Work out the finished part from the listing and answer in its coordinate system (mm). A direction names the side the tool comes from. Round coordinates to 2 decimals unless told otherwise and drop trailing zeros. Loops run counter-clockwise (first coordinate to the right, second up) from the corner with the lowest first, then second, coordinate; pieces in that order, holes last. Notation, with made-up numbers: M -8.5,18.25 L 25.5,18.25 A22 cw 25.5,55.25 Z; hole C 25.25,85 d10. An arc over 180 degrees is marked long. One line per item, written item: value.
```python
from build123d import *

# Parameters (mm, degrees)
BOSS_EXTRUDE1_DEPTH            = 8
CUT_EXTRUDE1_DEPTH             = 7
SKETCH3_R                      = 11
BOSS_EXTRUDE2_DEPTH            = 2
SKETCH4_R                      = 12.925
BOSS_EXTRUDE3_DEPTH            = 8
SKETCH5_R                      = 8.025
CUT_EXTRUDE2_DEPTH             = 31.757112998
SKETCH6_R                      = 6.125
CUT_EXTRUDE3_DEPTH             = 32.032241298
M8_CLEARANCE_HOLE1_D           = 9.25
M8_CLEARANCE_HOLE1_DEPTH       = 11
F_2_5_2_5_DIAMETER_HOLE1_D     = 2.5
F_2_5_2_5_DIAMETER_HOLE1_DEPTH = 10
FILLET1_R                      = 0.150000001
FILLET2_R                      = 0.5
CHAMFER1_SIZE                  = 0.5
CHAMFER1_SIZE2                 = 1
CHAMFER2_SIZE                  = 0.25
CHAMFER3_SIZE                  = 0.25


with BuildPart() as part:
    # Sketch1 → Boss-Extrude1 (new body)
    with BuildSketch(Plane.XZ):
        with BuildLine():
            Line((16.171038928, 21), (-16.171038928, 21))
            ThreePointArc((-16.171038928, 21), (-16.861657425, 20.876977915), (-17.467314594, 20.523046092))
            ThreePointArc((-17.467314594, 20.523046092), (-19.056527753, 19.056527753), (-20.523046092, 17.467314594))
            ThreePointArc((-20.523046092, 17.467314594), (-20.876977915, 16.861657425), (-21, 16.171038928))
            Line((-21, 16.171038928), (-21, -16.171038928))
            ThreePointArc((-21, -16.171038928), (-20.876977915, -16.861657425), (-20.523046092, -17.467314594))
            ThreePointArc((-20.523046092, -17.467314594), (-19.056527753, -19.056527753), (-17.467314594, -20.523046092))
            ThreePointArc((-17.467314594, -20.523046092), (-16.861657425, -20.876977915), (-16.171038928, -21))
            Line((-16.171038928, -21), (16.171038928, -21))
            ThreePointArc((16.171038928, -21), (16.861657424, -20.876977915), (17.467314593, -20.523046092))
            ThreePointArc((17.467314593, -20.523046092), (19.056527753, -19.056527753), (20.523046092, -17.467314593))
            ThreePointArc((20.523046092, -17.467314593), (20.876977914, -16.861657425), (21, -16.171038928))
            Line((21, -16.171038928), (21, 16.171038928))
            ThreePointArc((21, 16.171038928), (20.876977914, 16.861657425), (20.523046092, 17.467314593))
            ThreePointArc((20.523046092, 17.467314593), (19.056527753, 19.056527753), (17.467314593, 20.523046092))
            ThreePointArc((17.467314593, 20.523046092), (16.861657424, 20.876977915), (16.171038928, 21))
        make_face()
    extrude(amount=-BOSS_EXTRUDE1_DEPTH)

    # Sketch2 → Cut-Extrude1 (cut)
    with BuildSketch(Plane.XZ):
        Polygon((-19.5, 8.077164467), (-19.5, -8.077164467), (-8.077164467, -19.5), (8.077164467, -19.5), (19.5, -8.077164467), (19.5, 8.077164467), (8.077164467, 19.5), (-8.077164467, 19.5), align=None)
    extrude(amount=-CUT_EXTRUDE1_DEPTH, mode=Mode.SUBTRACT)

    # Sketch3 → Boss-Extrude2 (add)
    with BuildSketch(Plane(origin=(0, 8, 0), x_dir=(-1, 0, 0), z_dir=(0, 1, 0))):
        with Locations(Location((0, 0, 0), (0, 0, 270))):
            Circle(SKETCH3_R)
    extrude(amount=BOSS_EXTRUDE2_DEPTH)

    # Sketch4 → Boss-Extrude3 (add)
    with BuildSketch(Plane.XZ.offset(-7)):
        with Locations(Location((0, 0, 0), (0, 0, 270))):
            Circle(SKETCH4_R)
    extrude(amount=BOSS_EXTRUDE3_DEPTH)

    # Sketch5 → Cut-Extrude2 (cut, through all)
    with BuildSketch(Plane(origin=(0, 7, 0), x_dir=(1, 0, 0), z_dir=(0, 1, 0))):
        with Locations(Location((0, 0, 0), (0, 0, 90))):
            Circle(SKETCH5_R)
    extrude(amount=-CUT_EXTRUDE2_DEPTH, mode=Mode.SUBTRACT)

    # Sketch6 → Cut-Extrude3 (cut, through all)
    with BuildSketch(Plane(origin=(0, 8, 0), x_dir=(1, 0, 0), z_dir=(0, 1, 0))):
        with Locations(Location((0, 0, 0), (0, 0, 90))):
            Circle(SKETCH6_R)
    extrude(amount=-CUT_EXTRUDE3_DEPTH, mode=Mode.SUBTRACT)

    # M8 Clearance Hole1
    with Locations(Plane(origin=(0, 10, 0), x_dir=(1, 0, 0), z_dir=(0, 1, 0))):
        with Locations((0, 0)):
            Hole(M8_CLEARANCE_HOLE1_D / 2, depth=M8_CLEARANCE_HOLE1_DEPTH)

    # Ø2.5 (2.5) Diameter Hole1
    with Locations(Plane(origin=(0, 0, 0), x_dir=(-1, 0, 0), z_dir=(0, -1, 0))):
        with Locations((15.5, 15.5), (-15.5, -15.5), (-15.5, 15.5), (15.5, -15.5)):
            Hole(F_2_5_2_5_DIAMETER_HOLE1_D / 2, depth=F_2_5_2_5_DIAMETER_HOLE1_DEPTH)

    # Fillet1
    fillet1_edges = [part.edges().sort_by_distance(p)[0] for p in [
        (0, 8, 11),
        (0, 7, 12.925),
    ]]
    fillet(fillet1_edges, radius=FILLET1_R)

    # Fillet2
    fillet2_edges = [part.edges().sort_by_distance(p)[0] for p in [
        (-19.5, 3.5, 8.077164467),
        (-8.077164467, 3.5, 19.5),
        (8.077164467, 3.5, 19.5),
        (19.5, 3.5, 8.077164467),
        (19.5, 3.5, -8.077164467),
        (8.077164467, 3.5, -19.5),
        (-8.077164467, 3.5, -19.5),
        (-19.5, 3.5, -8.077164467),
    ]]
    fillet(fillet2_edges, radius=FILLET2_R)

    # Chamfer1
    chamfer1_edges = [part.edges().sort_by_distance(p)[0] for p in [
        (0, -1, 8.025),
    ]]
    chamfer1_side = [part.faces().sort_by_distance(p)[0] for p in [
        (0, -1, 12.559425794),
    ]]
    chamfer(chamfer1_edges, length=CHAMFER1_SIZE, length2=CHAMFER1_SIZE2, reference=chamfer1_side[0])

    # Chamfer2
    chamfer2_edges = [part.edges().sort_by_distance(p)[0] for p in [
        (16.861657424, 8, 20.876977915),
        (0, 8, 21),
        (-16.861657425, 8, 20.876977915),
        (-19.056527753, 8, 19.056527753),
        (-20.876977915, 8, 16.861657425),
        (-21, 8, 0),
        (-20.876977915, 8, -16.861657425),
        (-19.056527753, 8, -19.056527753),
        (-16.861657425, 8, -20.876977915),
        (0, 8, -21),
        (20.876977914, 8, 16.861657425),
        (16.861657424, 8, -20.876977915),
        (19.056527753, 8, -19.056527753),
        (20.876977914, 8, -16.861657425),
        (21, 8, 0),
        (19.056527753, 8, 19.056527753),
    ]]
    chamfer(chamfer2_edges, length=CHAMFER2_SIZE)

    # Chamfer3
    chamfer3_edges = [part.edges().sort_by_distance(p)[0] for p in [
        (0, 10, 11),
        (0, -1, 12.925),
        (0, 7, 6.125),
        (4.625, 10, 0),
    ]]
    chamfer(chamfer3_edges, length=CHAMFER3_SIZE)


solid = part.part
```
1) Find section A-A (y = 6.25). Give the number of separate pieces and of enclosed holes in the cut face, then the cut area to 3 significant figures.
Check values:
separate pieces: 2
enclosed holes: 6
area: 775 mm2
2) For faces 1 (the face through (-16.421, 4.056, -16.345)), 2 (the face through (13.711, 3.451, -13.866)), 3 (the face through (10.74, 8.94, 2.38)), determine the directions among +Z, -Z, +X, -X, +Y, -Y from which every point of the face is accessible in a straight line to the end or side of a thin tool.
Check values:
face 1: +Y, -Y
face 2: -Y
face 3: +Y
3) Each of these flat-tipped pins is pushed along its axis until it touches: pin 1 (10 mm diameter, centred on x = 2, z = 2, fed in from -Y); pin 2 (3 mm diameter, centred on x = -15.5, z = 15.5, fed in from -Y). Where does it stop, or does it pass through?
Check values:
pin 1: y = 7
pin 2: y = 0
4) Find section B-B (x = -15.5). Give the vertices of the cut face in (y, z).
Check values:
outline: M 0,-21 L 7.75,-21 L 8,-20.75 L 8,-16.75 L 0,-16.75 Z; M 0,-14.25 L 8,-14.25 L 8,14.25 L 0,14.25 L 0,12.08 L 7,12.08 L 7,-12.08 L 0,-12.08 Z; M 0,16.75 L 8,16.75 L 8,20.75 L 7.75,21 L 0,21 Z
5) Find section C-C (z = 15). Give the vertices of the cut face in (x, y).
Check values:
outline: M -21,0 L -16.65,0 L -16.65,8 L -20.75,8 L -21,7.75 Z; M -14.35,0 L -12.58,0 L -12.58,7 L 12.58,7 L 12.58,0 L 14.35,0 L 14.35,8 L -14.35,8 Z; M 16.65,0 L 21,0 L 21,7.75 L 20.75,8 L 16.65,8 Z
6) The mould has two halves that part along X. Classify faces 4 (the face through (-20.874, 3.821, 16.871)), 5 (the face through (-0.3, 7, 13.3)), 6 (the face through (14, 0, 14)): +X half, -X half, draft (parallel to the pull), parting line (faces both ways), or undercut.
Check values:
face 4: -X half
face 5: undercut
face 6: draft
7) Find the intervals of material crossed by probe 1 along X at (y, z) = (2.75, 0) (3 decimals); probe 2 along X at (y, z) = (4.75, 3.5); probe 3 along X at (y, z) = (2, 11), in increasing order. Write a range as from..to.
Check values:
probe 1: -21..-19.5, -12.925..-8.025, 8.025..12.925, 19.5..21
probe 2: -21..-19.5, -12.44..-7.22, 7.22..12.44, 19.5..21
probe 3: -21..-16.58, -6.79..6.79, 16.58..21
8) Find section D-D (y = 9.25). Give the vertices of the cut face in (x, z) (3 decimals).
Check values:
outline: C 0,0 d22; hole C 0,0 d9.25
